Could you check a few things on this model? Use its own coordinates, in mm. Give positions to 0.01 mm unless a question says otherwise; leave off trailing zeros. Loops run counter-clockwise (first coordinate to the right, second up) from the corner with the lowest first, then second, coordinate; pieces in that order, holes last. Notation, with made-up numbers: (-16.75, 2.25) -> (5.25, 2.25) arc R20 ccw to (5.25, 32.25) -> close; hole circle Ø4 at (-29, -25.75). An arc over 180 degrees is marked (long way). Put each result on its own line as item: value.
Autodesk Inventor part; units mm, degrees
ref_plane "YZ Plane" through (0, 0, 0) normal (1, 0, 0) x (0, 1, 0)
ref_plane "XZ Plane" through (0, 0, 0) normal (0, 1, 0) x (-1, 0, 0)
ref_plane "XY Plane" through (0, 0, 0) normal (0, 0, 1) x (1, 0, 0)
sketch "Sketch1" plane through (0, 0, 0) normal (0, 1, 0) x (-1, 0, 0)
  line L0 (0, 0) -> (0, -260)
  line L1 (0, -260) -> (47, -260)
  line L2 (47, -260) -> (47, -210)
  line L3 (47, -210) -> (50, -210)
  line L4 (47, -100) -> (50, -100)
  line L5 (50, -100) -> (50, -50)
  line L6 (50, -50) -> (47, -50)
  line L7 (47, -50) -> (47, 0)
  line L8 (47, 0) -> (0, 0)
  line L9 (47, -260) -> (50, -260) construction
  line L10 (47, -100) -> (47, -133)
  line L11 (47, -260) -> (36, -260) construction
  line L12 (36, -233) -> (17, -233)
  line L13 (17, -233) -> (17, -190)
  line L14 (17, -190) -> (20, -190)
  line L15 (47, -133) -> (35, -133) construction
  line L16 (35, -133) -> (35, -43)
  line L17 (35, -43) -> (22, -43)
  line L18 (22, -43) -> (22, -94)
  line L19 (22, -94) -> (16, -94)
  line L20 (16, -94) -> (16, -136)
  line L21 (16, -136) -> (20, -136)
  line L22 (20, -190) -> (20, -136)
  line L23 (47, -133) -> (35, -133)
  line L24 (50, -210) -> (50, -193)
  line L25 (36, -193) -> (50, -193)
  line L26 (36, -193) -> (36, -233)
  dimension "d0" = 260
  dimension "d1" = 47
  dimension "d2" = 50
  dimension "d3" = 3
  dimension "d6" = 50
  dimension "d10" = 11
  dimension "d14" = 19
  dimension "d15" = 12
  dimension "d16" = 90
  dimension "d17" = 13
  dimension "d18" = 51
  dimension "d19" = 6
  dimension "d20" = 42
  dimension "d24" = 67
  dimension "d25" = 60
extrude "Extrusion1" add sketch "Sketch1" along normal blind 3
properties part number "Atas Terminal"
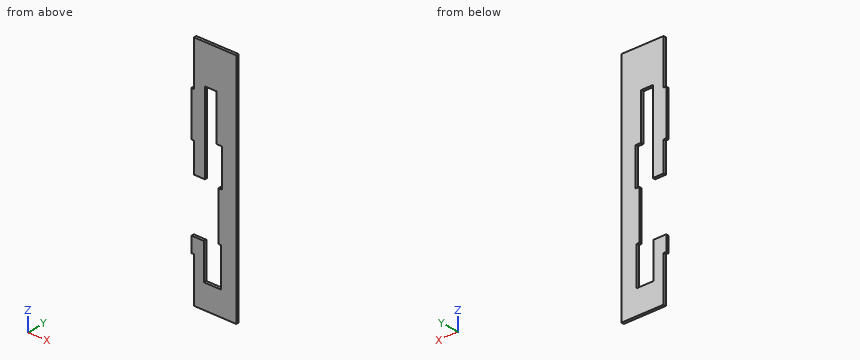
1. If we section it at C-C (y = 1.4): List the corners of the cut face in (x, z) for me.
Recorded:
outline: (-50, -210) -> (-47, -210) -> (-47, -260) -> (0, -260) -> (0, 0) -> (-47, 0) -> (-47, -50) -> (-50, -50) -> (-50, -100) -> (-47, -100) -> (-47, -133) -> (-35, -133) -> (-35, -43) -> (-22, -43) -> (-22, -94) -> (-16, -94) -> (-16, -136) -> (-20, -136) -> (-20, -190) -> (-17, -190) -> (-17, -233) -> (-36, -233) -> (-36, -193) -> (-50, -193) -> close
2. If we section it at B-B (x = -40): List the corners of the cut face in (y, z) for me, then the cut area to 3 significant figures.
Recorded:
outline: (0, -260) -> (3, -260) -> (3, -193) -> (0, -193) -> close; (0, -133) -> (3, -133) -> (3, 0) -> (0, 0) -> close
area: 600 mm^2
3. I need wall thicknesses on line 1 (Z direction, x = -17.5, y = 1.05); line 2 (X direction, y = 2.8, z = -197); line 3 (X direction, y = 0.8, z = -221.5). Which ranges of each line are inside material? Lowest first, please.
Recorded:
line 1: z = -260 to -233, -190 to -136, -94 to 0
line 2: x = -50 to -36, -17 to 0
line 3: x = -47 to -36, -17 to 0
4. If we section it at A-A (z = -202.5): List the corners of the cut face in (x, y) for me, then the cut area to 3 significant figures.
Recorded:
outline: (-50, 0) -> (-36, 0) -> (-36, 3) -> (-50, 3) -> close; (-17, 0) -> (0, 0) -> (0, 3) -> (-17, 3) -> close
area: 93.0 mm^2
5. If we section it at D-D (z = -20.5): List the corners of the cut face in (x, y) for me, then the cut area to 3 significant figures.
Recorded:
outline: (-47, 0) -> (0, 0) -> (0, 3) -> (-47, 3) -> close
area: 141 mm^2
6. I'm going to push flat-ended pins straight in: pin 1 (12 mm diameter, centred on x = -25.5, z = -206, fed in from -Y); pin 2 (0.9 mm diameter, centred on x = -48.5, y = 1.5, fed in from -Z); pin 3 (0.9 mm diameter, centred on y = 1.5, z = -119.5, fed in from -X). Where does each tip first touch, or does it pass through?
Recorded:
pin 1: passes through
pin 2: stops at z = -210
pin 3: stops at x = -47
